Could you check a few things on this model? Use its own coordinates, in mm. A direction names the side the tool comes from. Coordinates: 2 decimals unless noted, no trailing zeros. Order: outer loops, then holes, each group sorted by start corner. A loop starts at its lowest first (then second) coordinate and runs counter-clockwise, first axis right, second up. Notation, with made-up numbers: (-37.5, 59.25) -> (-23.5, 59.25) arc R14 cw to (-23.5, 75.25) -> close; hole circle Ø8 at (51.25, 73.5). An arc over 180 degrees is marked (long way). Put each result on its own line as item: value. Start each with the question number.
Q1. If we section it at C-C (x = 49): Please give me the cut outline in (y, z), and give its area (3 significant figures).
Q2. Will these pins go through, and if not, where does the flat tip stop? pin 1 (4 mm diameter, centred on y = 0, z = 16.5, fed in from +X); pin 2 (4 mm diameter, centred on x = -9.5, z = 22.5, fed in from +Y); pin 3 (8 mm diameter, centred on y = -14, z = 16.5, fed in from -X).
Q3. If we section it at B-B (z = 21): Please give me the cut outline in (x, y), and give its area (3 significant figures).
Q4. If we section it at D-D (x = 8): Please give me the cut outline in (y, z), and give its area (3 significant figures).
Q5. For faces 4 (the face through (38, 0, 4.75)), 5 (the face through (28, -25, 15)), 6 (the face through (-15.28, -11.71, 7.54)), which set-ups out of +Z, -Z, +X, -X, +Y, -Y let a thin tool reach every point of the face, with its end or its side?
Q6. We'd pull the mould along Y, two halves only. Please class faces 1 (the face through (-24.994, -0.55, 14.804)), 2 (the face through (55, 0, 2)), 3 (the face through (-8.8, -0.6, 2.5)): +Y half, -Y half, draft (parallel to the pull), parting line (faces both ways), or undercut.
Q7. Please list where these lines run through material, in increasing order: line 1 along Y through (x, z) = (45, 2); line 2 along Z through (x, y) = (48, -16.5); line 3 along Z through (x, y) = (-10.5, -15).
Q8. If we section it at A-A (z = 15): Please give me the cut outline in (x, y), and give its area (3 significant figures).
from build123d import *

# Parameters (mm, degrees)
BOSS_EXTRUDE2_DEPTH      = 30
SKETCH3_R                = 6.5
CUT_EXTRUDE2_DEPTH       = 40
SKETCH4_R                = 19
CUT_EXTRUDE3_DEPTH       = 25
SKETCH2_W                = 20.5
SKETCH2_H                = 40.5
CUT_EXTRUDE5_DEPTH       = 50
SKETCH6_R                = 6.75
CUT_EXTRUDE6_DEPTH       = 50
SKETCH7_R                = 19.25
CUT_EXTRUDE7_DEPTH       = 25
SKETCH8_W                = 30
SKETCH8_H                = 50
CUT_EXTRUDE8_DEPTH       = 15
CUT_EXTRUDE9_DEPTH       = 100
CUT_EXTRUDE9_DEPTH_BACK  = 15
SKETCH9_R                = 2
CUT_EXTRUDE10_DEPTH      = 100
CUT_EXTRUDE10_DEPTH_BACK = 15
SKETCH10_R               = 2
FILLET1_R                = 1
SKETCH12_R               = 6.75
SKETCH12_R_2             = 5
BOSS_EXTRUDE3_DEPTH      = 5
SKETCH13_R               = 1
CUT_EXTRUDE11_DEPTH      = 5
SKETCH14_R               = 19.25
SKETCH14_R_2             = 15
BOSS_EXTRUDE4_DEPTH      = 20


with BuildPart() as part:
    # Sketch1 → Boss-Extrude2 (new body)
    with BuildSketch(Plane.XY):
        with BuildLine():
            Line((0, 25), (70, 25))
            Line((70, 25), (70, -25))
            Line((70, -25), (0, -25))
            ThreePointArc((0, -25), (-25, 0), (0, 25))
        make_face()
    extrude(amount=BOSS_EXTRUDE2_DEPTH)

    # Sketch3 → Cut-Extrude2 (cut)
    with BuildSketch(Plane.XY.offset(30)):
        Circle(SKETCH3_R)
    extrude(amount=-CUT_EXTRUDE2_DEPTH, mode=Mode.SUBTRACT)

    # Sketch4 → Cut-Extrude3 (cut)
    with BuildSketch(Plane.XY.offset(30)):
        Circle(SKETCH4_R)
    extrude(amount=-CUT_EXTRUDE3_DEPTH, mode=Mode.SUBTRACT)

    # Sketch2 → Cut-Extrude5 (cut)
    with BuildSketch(Plane(origin=(70, 0, 0), x_dir=(0, 0, -1), z_dir=(1, 0, 0))):
        with Locations((-15, 0)):
            Rectangle(SKETCH2_W, SKETCH2_H)
    extrude(amount=-CUT_EXTRUDE5_DEPTH, mode=Mode.SUBTRACT)

    # Sketch6 → Cut-Extrude6 (cut)
    with BuildSketch(Plane.XY.offset(30)):
        Circle(SKETCH6_R)
    extrude(amount=-CUT_EXTRUDE6_DEPTH, mode=Mode.SUBTRACT)

    # Sketch7 → Cut-Extrude7 (cut)
    with BuildSketch(Plane.XY.offset(30)):
        Circle(SKETCH7_R)
    extrude(amount=-CUT_EXTRUDE7_DEPTH, mode=Mode.SUBTRACT)

    # Sketch8 → Cut-Extrude8 (cut)
    with BuildSketch(Plane(origin=(70, 0, 0), x_dir=(0, 0, -1), z_dir=(1, 0, 0))):
        with Locations((-15, 0)):
            Rectangle(SKETCH8_W, SKETCH8_H)
    extrude(amount=-CUT_EXTRUDE8_DEPTH, mode=Mode.SUBTRACT)

    # Sketch9 → Cut-Extrude9 (cut, two sides: drawn at the far end of the back side and taken through both)
    with BuildSketch(Plane.XY.offset(4.75).offset(-CUT_EXTRUDE9_DEPTH_BACK)):
        with Locations(Location((45, -10.25, 0), (0, 0, 180))):
            Circle(SKETCH9_R)
        with Locations(Location((45, 9.75, 0), (0, 0, 180))):
            Circle(SKETCH9_R)
    extrude(amount=CUT_EXTRUDE9_DEPTH + CUT_EXTRUDE9_DEPTH_BACK, mode=Mode.SUBTRACT)

    # Sketch10 → Cut-Extrude10 (cut, two sides: drawn at the far end of the back side and taken through both)
    with BuildSketch(Plane(origin=(0, -20.25, 0), x_dir=(1, 0, 0), z_dir=(0, 1, 0)).offset(-CUT_EXTRUDE10_DEPTH_BACK)):
        with Locations(Location((45, -15, 0), (0, 0, 90))):
            Circle(SKETCH10_R)
    extrude(amount=CUT_EXTRUDE10_DEPTH + CUT_EXTRUDE10_DEPTH_BACK, mode=Mode.SUBTRACT)

    # Fillet1
    fillet1_edges = [part.edges().sort_by_distance(p)[0] for p in [
        (-25, 0, 30),
        (27.5, -25, 0),
        (27.5, 25, 0),
        (27.5, 25, 30),
        (-25, 0, 0),
        (27.5, -25, 30),
    ]]
    fillet(fillet1_edges, radius=FILLET1_R)

    # Sketch12 → Boss-Extrude3 (add)
    with BuildSketch(Plane.XY.offset(5)):
        Circle(SKETCH12_R)
        Circle(SKETCH12_R_2, mode=Mode.SUBTRACT)
    extrude(amount=-BOSS_EXTRUDE3_DEPTH)

    # Sketch13 → Cut-Extrude11 (cut)
    with BuildSketch(Plane.XY.offset(5)):
        with Locations((-8, 0)):
            Circle(SKETCH13_R)
        with Locations((0, 8)):
            Circle(SKETCH13_R)
        with Locations((8, 0)):
            Circle(SKETCH13_R)
        with Locations((0, -8)):
            Circle(SKETCH13_R)
    extrude(amount=-CUT_EXTRUDE11_DEPTH, mode=Mode.SUBTRACT)

    # Sketch14 → Boss-Extrude4 (add)
    with BuildSketch(Plane.XY.offset(30)):
        Circle(SKETCH14_R)
        Circle(SKETCH14_R_2, mode=Mode.SUBTRACT)
    extrude(amount=-BOSS_EXTRUDE4_DEPTH)


solid = part.part
The answers:
1. outline: (-25, 1) arc R1 ccw to (-24, 0) -> (24, 0) arc R1 ccw to (25, 1) -> (25, 29) arc R1 ccw to (24, 30) -> (-24, 30) arc R1 ccw to (-25, 29) -> close; hole (-20.25, 4.75) -> (20.25, 4.75) -> (20.25, 25.25) -> (-20.25, 25.25) -> close
1. area: 669 mm^2
2. pin 1: x = 20
2. pin 2: y = 23.85
2. pin 3: x = -22.91
3. outline: (0, -25) -> (55, -25) -> (55, -20.25) -> (20, -20.25) -> (20, 20.25) -> (55, 20.25) -> (55, 25) -> (0, 25) arc R25 ccw to start; hole circle Ø30 at (0, 0)
3. area: 1,610 mm^2
4. outline: (-25, 1) arc R1 ccw to (-24, 0) -> (-1, 0) -> (-1, 5) -> (-17.51, 5) -> (-17.51, 10) -> (-12.69, 10) -> (-12.69, 30) -> (-24, 30) arc R1 ccw to (-25, 29) -> close; (1, 0) -> (24, 0) arc R1 ccw to (25, 1) -> (25, 29) arc R1 ccw to (24, 30) -> (12.69, 30) -> (12.69, 10) -> (17.51, 10) -> (17.51, 5) -> (1, 5) -> close
4. area: 807 mm^2
5. face 4: +X
5. face 5: +Z, -Z, +X, -X, -Y
5. face 6: none
6. face 1: parting line
6. face 2: draft
6. face 3: undercut
7. line 1: -25 to -12.25, -8.25 to 7.75, 11.75 to 25
7. line 2: 0 to 4.75, 25.25 to 30
7. line 3: 0 to 5, 10 to 30
8. outline: (0, -25) -> (43, -25) -> (43, -20.25) -> (20, -20.25) -> (20, 20.25) -> (43, 20.25) -> (43, 25) -> (0, 25) arc R25 ccw to start; (47, -25) -> (55, -25) -> (55, -20.25) -> (47, -20.25) -> close; (47, 20.25) -> (55, 20.25) -> (55, 25) -> (47, 25) -> close; hole circle Ø30 at (0, 0)
8. area: 1,570 mm^2
